```python
from build123d import *

# Parameters (mm, degrees)
BOSS_EXTRUDE1_DEPTH = 1.6
CUT_EXTRUDE1_DEPTH  = 1.6


with BuildPart() as part:
    # Sketch2 → Boss-Extrude1 (new body)
    with BuildSketch(Plane.XY):
        Polygon((5193.573840828, 1803.237079941), (5212.573840828, 1803.237079941), (5212.573840828, 1812.937079941), (5285.973840828, 1812.937079941), (5285.973840828, 1803.237079941), (5304.973840828, 1803.237079941), (5304.973840828, 1631.237079941), (5285.973840828, 1631.237079941), (5285.973840828, 1621.537079941), (5212.573840828, 1621.537079941), (5212.573840828, 1631.237079941), (5193.573840828, 1631.237079941), align=None)
    extrude(amount=BOSS_EXTRUDE1_DEPTH)

    # Sketch3 → Cut-Extrude1 (cut)
    with BuildSketch(Plane.XY.offset(1.6)):
        with BuildLine():
            ThreePointArc((5202.323840828, 1797.736928772), (5203.973840828, 1796.086928772), (5205.623840828, 1797.736928772))
            ThreePointArc((5205.623840828, 1797.736928772), (5203.973840828, 1799.386928772), (5202.323840828, 1797.736928772))
        make_face()
        with BuildLine():
            ThreePointArc((5296.223840828, 1797.736928772), (5294.573840828, 1799.386928772), (5292.923840828, 1797.736928772))
            ThreePointArc((5292.923840828, 1797.736928772), (5294.573840828, 1796.086928772), (5296.223840828, 1797.736928772))
        make_face()
        with BuildLine():
            ThreePointArc((5296.223840828, 1636.736928772), (5294.573840828, 1638.386928772), (5292.923840828, 1636.736928772))
            ThreePointArc((5292.923840828, 1636.736928772), (5294.573840828, 1635.086928772), (5296.223840828, 1636.736928772))
        make_face()
        with BuildLine():
            ThreePointArc((5205.623840828, 1636.736928772), (5203.973840828, 1638.386928772), (5202.323840828, 1636.736928772))
            ThreePointArc((5202.323840828, 1636.736928772), (5203.973840828, 1635.086928772), (5205.623840828, 1636.736928772))
        make_face()
    extrude(amount=-CUT_EXTRUDE1_DEPTH, mode=Mode.SUBTRACT)


solid = part.part
```
The listing builds one solid part. Answer for the finished solid, in the listing's coordinates (mm). Round coordinates to 2 decimals unless told otherwise and drop trailing zeros. Loops run counter-clockwise (first coordinate to the right, second up) from the corner with the lowest first, then second, coordinate; pieces in that order, holes last.
Q1. Section A-A, the plane z = 0.25 is taken. Determine the outline of the cut face in (x, y), then the cut area to 3 significant figures.
Q2. Find the intervals of material crossed by line 1 (Y direction, x = 5299.5, z = 0.35), in increasing order.
Q3. Given pin 1 Ø0.5 at (y, z) = (1625.5, 0.5) entering from -X; pin 2 Ø0.5 at (y, z) = (1809.5, 1) entering from +X; pin 3 Ø2 at (x, y) = (5203.97, 1636.74) entering from -Z, each flat-ended and moving along its own axis, determine where each tip first touches the part or whether it passes through.
Completed:
1. outline: (5193.57, 1631.24) - (5212.57, 1631.24) - (5212.57, 1621.54) - (5285.97, 1621.54) - (5285.97, 1631.24) - (5304.97, 1631.24) - (5304.97, 1803.24) - (5285.97, 1803.24) - (5285.97, 1812.94) - (5212.57, 1812.94) - (5212.57, 1803.24) - (5193.57, 1803.24) - close; hole circle Ø3.3 at (5203.97, 1636.74); hole circle Ø3.3 at (5203.97, 1797.74); hole circle Ø3.3 at (5294.57, 1636.74); hole circle Ø3.3 at (5294.57, 1797.74)
1. area: 20,600 mm2
2. line 1: y = 1631.24 to 1803.24
3. pin 1: stops at x = 5212.57
3. pin 2: stops at x = 5285.97
3. pin 3: passes through
